```python
from build123d import *

# Parameters (mm, degrees)
EXTRUDE_1_DEPTH     = 30
SKETCH_2_W          = 5
SKETCH_2_H          = 54
CUT_EXTRUDE_1_DEPTH = 45
FILLET_1_R          = 1
SKETCH_4_R          = 3
CUT_EXTRUDE_2_DEPTH = 45
SKETCH_5_R          = 2.5
CUT_EXTRUDE_3_DEPTH = 92
FILLET_2_R          = 1.2


with BuildPart() as part:
    # 草图1 → 凸台-拉伸1 (new body)
    with BuildSketch(Plane(origin=(0, 0, 0), x_dir=(0, 0, -1), z_dir=(1, 0, 0))):
        Polygon((0, 30), (0, 0), (-33, 0), (-3, 30), align=None)
    extrude(amount=EXTRUDE_1_DEPTH)

    # 草图2 → 切除-拉伸1 (cut)
    with BuildSketch(Plane(origin=(0, 0, 3), x_dir=(-1, 0, 0), z_dir=(0, 0, -1))):
        with BuildLine():
            Line((-19.5, 15), (-19.5, 31.772972214))
            ThreePointArc((-19.5, 31.772972214), (-15, 36.272972214), (-10.5, 31.772972214))
            Line((-10.5, 31.772972214), (-10.5, 15))
            ThreePointArc((-10.5, 15), (-15, 10.5), (-19.5, 15))
        make_face()
        with Locations((-5.5, 30)):
            Rectangle(SKETCH_2_W, SKETCH_2_H)
        with Locations((-24.5, 30)):
            Rectangle(SKETCH_2_W, SKETCH_2_H)
    extrude(amount=-CUT_EXTRUDE_1_DEPTH, mode=Mode.SUBTRACT)

    # 圆角1
    fillet_1_edges = [part.edges().sort_by_distance(p)[0] for p in [
        (27, 3, 16.5),
        (22, 3, 16.5),
        (8, 3, 16.5),
        (3, 3, 16.5),
    ]]
    fillet(fillet_1_edges, radius=FILLET_1_R)

    # 草图4 → 切除-拉伸2 (cut)
    with BuildSketch(Plane.XY.offset(3)):
        with Locations((15, 15)):
            Circle(SKETCH_4_R)
    extrude(amount=-CUT_EXTRUDE_2_DEPTH, mode=Mode.SUBTRACT)

    # 草图5 → 切除-拉伸3 (cut)
    with BuildSketch(Plane.XY):
        with Locations((15, 6)):
            Circle(SKETCH_5_R)
    extrude(amount=CUT_EXTRUDE_3_DEPTH, mode=Mode.SUBTRACT)

    # 圆角2
    fillet_2_edges = [part.edges().sort_by_distance(p)[0] for p in [
        (30, 0, 16.5),
        (30, 30, 1.5),
        (0, 0, 16.5),
        (0, 30, 1.5),
    ]]
    fillet(fillet_2_edges, radius=FILLET_2_R)


solid = part.part
```
Verification items for the finished model (mm, model axes). A direction names the side the tool comes from. Coordinates: 2 decimals unless noted, no trailing zeros. Order: outer loops, then holes, each group sorted by start corner. A loop starts at its lowest first (then second) coordinate and runs counter-clockwise, first axis right, second up. Notation, with made-up numbers: (-33, 20) - (-16, 20) arc R22 cw to (-16, 43) - close; hole circle Ø11 at (69.25, 69). An arc over 180 degrees is marked (long way). Return JSON: item names as keys, results as strings.
(1) Section check B-B, the plane z = 11. Record the cut outline in (x, y), and give its area (3 significant figures).
Filled sheet:
{"outline": "(0, 1.2) arc R1.2 ccw to (1.2, 0) - (28.8, 0) arc R1.2 ccw to (30, 1.2) - (30, 22) - (27, 22) - (27, 4) arc R1 cw to (26, 3) - (23, 3) arc R1 cw to (22, 4) - (22, 22) - (19.5, 22) - (19.5, 15) arc R4.5 cw to (10.5, 15) - (10.5, 22) - (8, 22) - (8, 4) arc R1 cw to (7, 3) - (4, 3) arc R1 cw to (3, 4) - (3, 22) - (0, 22) - close; hole circle Ø5 at (15, 6)", "area": "356 mm^2"}
(2) Section check C-C, the plane x = 15. Record the cut outline in (y, z), and give its area (3 significant figures).
Filled sheet:
{"outline": "(0, 0) - (3.5, 0) - (3.5, 29.5) - (0, 33) - close; (8.5, 0) - (12, 0) - (12, 3) - (10.5, 3) - (10.5, 22.5) - (8.5, 24.5) - close; (18, 0) - (30, 0) - (30, 3) - (18, 3) - close", "area": "197 mm^2"}
(3) Mould release check, pull along Y, two halves, no side actions. Record for faces 3 (the cylindrical face through (12.6, 13.2, 1.5)), 4 (the cylindrical face through (7.699, 3.285, 16.689)), 5 (the flat face through (6, 17, 3)): pulls with the +Y half, pulls with the -Y half, needs draft (parallel to the pull), parting line crosses it, or undercut.
Filled sheet:
{"face 3": "undercut", "face 4": "pulls with the +Y half", "face 5": "needs draft"}
(4) Section check D-D, the plane y = 25. Record the cut outline in (x, z), and give its area (3 significant figures).
Filled sheet:
{"outline": "(0, 0) - (30, 0) - (30, 8) - (27, 8) - (27, 3) - (22, 3) - (22, 8) - (19.5, 8) - (19.5, 3) - (10.5, 3) - (10.5, 8) - (8, 8) - (8, 3) - (3, 3) - (3, 8) - (0, 8) - close", "area": "145 mm^2"}
(5) Go/stop test with flat-tipped pins: pin 1 (2.5 mm diameter, centred on x = 13.5, y = 18, fed in from +Z); pin 2 (0.9 mm diameter, centred on x = 5.5, z = 17, fed in from +Y); pin 3 (4 mm diameter, centred on x = 23.5, y = 10, fed in from +Z); pin 4 (9.5 mm diameter, centred on x = 15, y = 15, fed in from -Z). Record where each tip stops, or that it passes through.
Filled sheet:
{"pin 1": "stops at z = 3", "pin 2": "stops at y = 3", "pin 3": "stops at z = 24.32", "pin 4": "stops at z = 0"}
(6) Thickness scan on line 1 along X through (y, z) = (6, 12); line 2 along X through (y, z) = (10, 13.5); line 3 along Y through (x, z) = (15, 0.75). Record the ranges inside material, lowest first.
Filled sheet:
{"line 1": "x = 0 to 3, 8 to 12.5, 17.5 to 22, 27 to 30", "line 2": "x = 0 to 3, 8 to 22, 27 to 30", "line 3": "y = 0 to 3.5, 8.5 to 12, 18 to 30"}
(7) Access from +Z, -Z, +X, -X, +Y, -Y to the whole of each face (thin tool, end or side, straight path). Record for faces 1 (the cylindrical face through (0.342, 0.361, 16.731)), 2 (the flat face through (27, 14, 13)).
Filled sheet:
{"face 1": "+Z, -Z, -X, -Y", "face 2": "+Z, +Y"}
(8) Section check A-A, the plane y = 6. Record the cut outline in (x, z), and give its area (3 significant figures).
Filled sheet:
{"outline": "(0, 0) - (12.5, 0) - (12.5, 27) - (8, 27) - (8, 3) - (3, 3) - (3, 27) - (0, 27) - close; (17.5, 0) - (30, 0) - (30, 27) - (27, 27) - (27, 3) - (22, 3) - (22, 27) - (17.5, 27) - close", "area": "435 mm^2"}
